```python
from build123d import *

# Parameters (mm, degrees)
F0_W     = 22.5
F0_H     = 8
F2_DEPTH = 3
F1_W     = 22.5
F1_H     = 2
F3_DEPTH = 1
F5_D     = 6.1
F6_R     = 0.748406
F7_R     = 0.748


with BuildPart() as f2:
    # F0 (on Front) → F2 (new body)
    with BuildSketch(Plane.XZ):
        Rectangle(F0_W, F0_H)
    extrude(amount=F2_DEPTH)

    # F1 (on Front) → F3 (join)
    with BuildSketch(Plane.XZ):
        Rectangle(F1_W, F1_H)
    extrude(amount=-F3_DEPTH)

    # F5 (through all)
    with Locations(Plane.XZ.offset(3)):
        with Locations((-5.941246, 0)):
            Hole(F5_D / 2)

    # F6
    f6_edges = [f2.edges().sort_by_distance(p)[0] for p in [
        (-11.25, 1, 0),
    ]]
    fillet(f6_edges, radius=F6_R)

    # F7
    f7_edges = [f2.edges().sort_by_distance(p)[0] for p in [
        (11.25, 1, 0),
    ]]
    fillet(f7_edges, radius=F7_R)


solid = f2.part
```
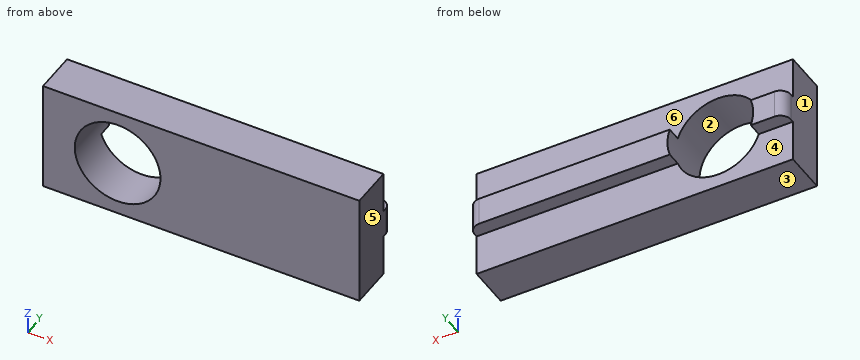
The listing builds one solid part. Answer for the finished solid, in the listing's coordinates (mm). Face numbers are marked on the shaded views. A direction names the side the tool comes from. Coordinates: 2 decimals unless noted, no trailing zeros. Write each loop counter-clockwise with the first axis right and the second up, starting at its lowest first coordinate (ties: lowest second). Pieces come first, ordered by that corner, then holes. Notation, with made-up numbers: (41.25, 82.5) - (65.25, 82.5) arc R16 ccw to (65.25, 95.5) - close; hole circle Ø1 at (55, -11.75). An arc over 180 degrees is marked (long way). One line per item, written item: value.
1) Find section A-A (z = 0). Give the vertices of the cut face in (x, y).
Geometry check:
outline: (-11.25, -3) - (-8.99, -3) - (-8.99, 1) - (-10.5, 1) arc R0.75 ccw to (-11.25, 0.25) - close; (-2.89, -3) - (11.25, -3) - (11.25, 0.25) arc R0.75 ccw to (10.5, 1) - (-2.89, 1) - close
2) A tool of negligible diameter and unlimited length cuts with its end or side. For the marked faces 4, 5 and 6, from which of +Z, -Z, +X, -X, +Y, -Y can it reach the whole face along a straight path? Write none if from no direction.
Geometry check:
face 4: -Z, +X, -X, +Y
face 5: +Z, -Z, +X, +Y, -Y
face 6: +Z, +X, -X, +Y
3) For a pull along X with two mould halves and no side action, classify the marked faces 1, 2 and 3 as pulls with the +X half, pulls with the -X half, needs draft (parallel to the pull), parting line crosses it, or undercut.
Geometry check:
face 1: pulls with the -X half
face 2: undercut
face 3: needs draft
4) Consider line 1 along X through (y, z) = (-0.95, 0); line 2 along Z through (x, y) = (-6, -2.15); line 3 along Y through (x, z) = (-1.5, 1.25). Determine where each line is inside the solid, lowest interval first. Write a range as from..to.
Geometry check:
line 1: x = -11.25..-8.99, -2.89..11.25
line 2: z = -4..-3.05, 3.05..4
line 3: y = -3..0
5) Find section D-D (x = -4.75). Give the vertices of the cut face in (y, z), and give its area (3 significant figures).
Geometry check:
outline: (-3, -4) - (0, -4) - (0, -2.81) - (-3, -2.81) - close; (-3, 2.81) - (0, 2.81) - (0, 4) - (-3, 4) - close
area: 7.15 mm2
6) Each of these flat-tipped pins is pushed along its axis until it touches: pin 1 Ø0.5 at (x, y) = (-10, 0.5) entering from +Z; pin 2 Ø1.5 at (x, z) = (-5.5, -2.5) entering from +Y; pin 3 Ø3.5 at (x, z) = (-5.94, 0) entering from -Y (3 decimals). Where does it stop, or does it pass through?
Geometry check:
pin 1: stops at z = 1
pin 2: stops at y = 0
pin 3: passes through
7) Find section B-B (y = -2.35). Give the vertices of the cut face in (x, z).
Geometry check:
outline: (-11.25, -4) - (11.25, -4) - (11.25, 4) - (-11.25, 4) - close; hole circle Ø6.1 at (-5.94, 0)
8) Find section C-C (x = 7.75). Give the vertices of the cut face in (y, z), and give its area (3 significant figures).
Geometry check:
outline: (-3, -4) - (0, -4) - (0, -1) - (1, -1) - (1, 1) - (0, 1) - (0, 4) - (-3, 4) - close
area: 26.0 mm2
